from build123d import *

# Parameters (mm, degrees)
SKETCH3_R          = 4.7625
CUT_EXTRUDE1_DEPTH = 66.838201297


with BuildPart() as part:
    # Sketch2 → Revolve1 (revolve)
    with BuildSketch(Plane.XY, mode=Mode.PRIVATE) as revolve1_sk:
        Polygon((2.040850661, 44.45), (0, 42.017808893), (0, 0), (2.2225, 0), (2.2225, 12.7), (12.7, 12.7), (12.7, 57.15), (-3.175, 57.15), (-3.175, 47.625), (9.525, 47.625), (9.525, 44.45), align=None)
    revolve(revolve1_sk.sketch.rotate(Axis((12.7, 12.7, 0), (0, 1, 0)), 270), axis=Axis((12.7, 12.7, 0), (0, 1, 0)))

    # Sketch3 → Cut-Extrude1 (cut, through all)
    with BuildSketch(Plane.XY):
        with Locations((12.7, 25.4)):
            Circle(SKETCH3_R)
    extrude(amount=-CUT_EXTRUDE1_DEPTH, mode=Mode.SUBTRACT)


solid = part.part
Read the model definition and answer for the solid it produces. Units are mm, in the model's axes. A direction names the side the tool comes from. Give positions to 0.01 mm unless a question says otherwise; leave off trailing zeros. Write each loop counter-clockwise with the first axis right and the second up, starting at its lowest first coordinate (ties: lowest second). Pieces come first, ordered by that corner, then holes. Notation, with made-up numbers: (-18, -2.5) -> (24, -2.5) arc R19 ccw to (24, 29.5) -> close; hole circle Ø3 at (57, 32.5). An arc over 180 degrees is marked (long way). Answer as a JSON object with one key per item and string values. Group by question number.
1) Find section D-D (y = 20). Write down the section's boundary in (x, z), and give its area (3 significant figures).
2) Find section C-C (y = 12). Write down the section's boundary in (x, z) (1 decimal), and give its area (3 significant figures).
3) The mould has two halves that part along Y. Classify faces 5 (the conical face through (23.23, 44.3, 2.34)), 6 (the flat face through (2, 0, -2)), 7 (the cylindrical face through (15.8, 46.02, 0.69)), 8 (the cylindrical face through (2.31, 6.44, 1.36)): +Y half, -Y half, draft (parallel to the pull), parting line (faces both ways), or undercut.
4) A tool of negligible diameter and unlimited length cuts with its end or side. For faces 1 (the cylindrical face through (20.4, 20.7, 10.1)), 2 (the cylindrical face through (11.67, 20.75, -6.26)), 3 (the cylindrical face through (7.93, 52.32, -15.14)), 4 (the flat face through (15, 44.45, -3)), from which of +Z, -Z, +X, -X, +Y, -Y can it reach the whole face along a straight path? Write none if from no direction.
5) Consider L1, parallel to Y at x = 7, z = 0.5 (3 decimals); L2, parallel to Y at x = 12, z = -4 (3 decimals); L3, parallel to Y at x = 17, z = -2 (3 decimals). Determine where each line is inside the solid, lowest interval first. Write a range as from..to.
6) Find section B-B (z = -6). Count the separate pieces of the cut face and the enclosed holes in it, and give its area (3 significant figures).
7) Each of these flat-tipped pins is pushed along its axis until it touches: P1, Ø1, axis at y = 28.5, z = -4.5, coming from the -X side; P2, Ø11, axis at x = 12.7, y = 25.4, coming from the -Z side; P3, Ø5, axis at x = 7.5, y = 26.5, coming from the -Z side. Where does it stop, or does it pass through?
Values follow:
{
 "1": {"outline": "circle Ø25.4 at (12.7, 0)", "area": "507 mm2"},
 "2": {"outline": "circle Ø25.4 at (12.7, 0); hole circle Ø21 at (12.7, 0)", "area": "162 mm2"},
 "3": {"face 5": "undercut", "face 6": "-Y half", "face 7": "undercut", "face 8": "draft"},
 "4": {"face 1": "-Y", "face 2": "-Z", "face 3": "+Y, -Y", "face 4": "none"},
 "5": {"L1": "y = 12.7..44.45, 47.625..57.15", "L2": "y = 12.7..20.689, 30.111..44.45, 47.625..57.15", "L3": "y = 12.7..23.353, 27.447..44.45, 47.625..57.15"},
 "6": {"separate pieces": "2", "enclosed holes": "1", "area": "980 mm2"},
 "7": {"P1": "stops at x = 0.65", "P2": "stops at z = -12.7", "P3": "stops at z = -12.16"}
}
